Check sheet for the modelled part. Datum: model origin and axes. Units: mm. Round coordinates to 2 decimals unless told otherwise and drop trailing zeros. Loops run counter-clockwise (first coordinate to the right, second up) from the corner with the lowest first, then second, coordinate; pieces in that order, holes last. Notation, with made-up numbers: (-30, -3) - (6, -3) arc R24 ccw to (6, 10) - close; hole circle Ø5 at (65.25, 78). An arc over 180 degrees is marked (long way). Put each result on its own line as item: value. Start each with the question number.
Item 1: Draft check along Z on faces 1 (the flat face through (-71, 0, -56)), 2 (the cylindrical face through (-93.08, 1.01, -87.19)). Enter one of: pulls with the +Z half, pulls with the -Z half, needs draft (parallel to the pull), parting line crosses it, or undercut.
Item 2: Material ranges on line 1 along X through (y, z) = (1.3, -89.5); line 2 along X through (y, z) = (0.4, -105); line 3 along X through (y, z) = (1.3, -90), recorded low to high.
Item 3: Section check D-D, the plane y = 1.3. Give the number of separate pieces and of enclosed holes in the cut face, and give its area (3 significant figures).
Item 4: Section check B-B, the plane z = -90. Record the cut outline in (x, y), and give its area (3 significant figures).
Item 5: Section check A-A, the plane x = -5. Record the cut outline in (y, z), and give its area (3 significant figures).
Item 6: Section check C-C, the plane z = -105. Record the cut outline in (x, y), and give its area (3 significant figures).
Item 7: Gauge pin test, flat ends, axial feed: pin 1 Ø5.5 at (x, z) = (-135, -105) entering from +Y; pin 2 Ø4 at (x, z) = (-70, -105) entering from +Y. Record the tip position at first contact, or that the pin passes through.
from build123d import *

# Parameters (mm, degrees)
BOTTOM_PLATE_W                       = 140
BOTTOM_PLATE_H                       = 110
BOTTOM_PLATE_EXT_DEPTH               = 2
MIDDLE_ROW_R                         = 6
MIDDLE_ROW_CUT_DEPTH                 = 179.056170912
TOP_ROW_R                            = 6.1
TOP_ROW_CUT_DEPTH                    = 179.056170912
BOTTOM_ROW_R                         = 3.55
BOTTOM_ROW_R_2                       = 6
BOTTOM_ROW_CUT_DEPTH                 = 179.056170912
PLATE_SCREWS_R                       = 1.65
PLATE_SCREWS_CUT_DEPTH               = 179.056170912
PLATE_SCREW_HEAD_R                   = 2.8
PLATE_SCREW_HEAD_CUT_DEPTH           = 2
PLATE_SCREW_HEAD_CUT_DRAFT           = -45
PLATE_SCREW_HEAD_CUT_PROFILE_2_DEPTH = 2
PLATE_SCREW_HEAD_CUT_PROFILE_2_DRAFT = -45
PLATE_SCREW_HEAD_CUT_PROFILE_3_DEPTH = 2
PLATE_SCREW_HEAD_CUT_PROFILE_3_DRAFT = -45
PLATE_SCREW_HEAD_CUT_PROFILE_4_DEPTH = 2
PLATE_SCREW_HEAD_CUT_PROFILE_4_DRAFT = -45
PLATE_SCREW_HEAD_CUT_PROFILE_5_DEPTH = 2
PLATE_SCREW_HEAD_CUT_PROFILE_5_DRAFT = -45
PLATE_SCREW_HEAD_CUT_PROFILE_6_DEPTH = 2
PLATE_SCREW_HEAD_CUT_PROFILE_6_DRAFT = -45
FILLET1_R                            = 2
FILLET2_R                            = 2
FILLET3_R                            = 2
FILLET4_R                            = 2


with BuildPart() as part:
    # Bottom Plate → Bottom Plate EXT (new body)
    with BuildSketch(Plane(origin=(0, 0, 0), x_dir=(1, 0, 0), z_dir=(0, 1, 0))):
        with Locations((-70, 55)):
            Rectangle(BOTTOM_PLATE_W, BOTTOM_PLATE_H)
    extrude(amount=BOTTOM_PLATE_EXT_DEPTH)

    # Middle Row → Middle Row Cut (cut, through all)
    with BuildSketch(Plane(origin=(0, 2, 0), x_dir=(1, 0, 0), z_dir=(0, 1, 0))):
        with Locations(Location((-123, 55, 0), (0, 0, 270))):
            Circle(MIDDLE_ROW_R)
        with Locations(Location((-87.666666667, 55, 0), (0, 0, 270))):
            Circle(MIDDLE_ROW_R)
        with Locations(Location((-52.333333333, 55, 0), (0, 0, 270))):
            Circle(MIDDLE_ROW_R)
        with Locations(Location((-17, 55, 0), (0, 0, 270))):
            Circle(MIDDLE_ROW_R)
    extrude(amount=-MIDDLE_ROW_CUT_DEPTH, mode=Mode.SUBTRACT)

    # Top Row → Top Row Cut (cut, through all)
    with BuildSketch(Plane(origin=(0, 2, 0), x_dir=(1, 0, 0), z_dir=(0, 1, 0))):
        with Locations(Location((-123, 90, 0), (0, 0, 270))):
            Circle(TOP_ROW_R)
        with Locations(Location((-87.666666667, 90, 0), (0, 0, 270))):
            Circle(TOP_ROW_R)
        with Locations(Location((-52.333333333, 90, 0), (0, 0, 270))):
            Circle(TOP_ROW_R)
        with Locations(Location((-17, 90, 0), (0, 0, 270))):
            Circle(TOP_ROW_R)
    extrude(amount=-TOP_ROW_CUT_DEPTH, mode=Mode.SUBTRACT)

    # Bottom Row → Bottom Row Cut (cut, through all)
    with BuildSketch(Plane(origin=(0, 2, 0), x_dir=(1, 0, 0), z_dir=(0, 1, 0))):
        with Locations(Location((-87.666666667, 20, 0), (0, 0, 270))):
            Circle(BOTTOM_ROW_R)
        with Locations(Location((-52.333333333, 20, 0), (0, 0, 270))):
            Circle(BOTTOM_ROW_R)
        with Locations(Location((-17, 20, 0), (0, 0, 270))):
            Circle(BOTTOM_ROW_R)
        with Locations(Location((-123, 20, 0), (0, 0, 270))):
            Circle(BOTTOM_ROW_R_2)
    extrude(amount=-BOTTOM_ROW_CUT_DEPTH, mode=Mode.SUBTRACT)

    # Plate Screws → Plate Screws Cut (cut, through all)
    with BuildSketch(Plane(origin=(0, 2, 0), x_dir=(1, 0, 0), z_dir=(0, 1, 0))):
        with Locations(Location((-135, 105, 0), (0, 0, 270))):
            Circle(PLATE_SCREWS_R)
        with Locations(Location((-5, 105, 0), (0, 0, 270))):
            Circle(PLATE_SCREWS_R)
        with Locations(Location((-5, 5, 0), (0, 0, 270))):
            Circle(PLATE_SCREWS_R)
        with Locations(Location((-135, 5, 0), (0, 0, 270))):
            Circle(PLATE_SCREWS_R)
        with Locations(Location((-70, 105, 0), (0, 0, 270))):
            Circle(PLATE_SCREWS_R)
        with Locations(Location((-70, 5, 0), (0, 0, 90))):
            Circle(PLATE_SCREWS_R)
    extrude(amount=-PLATE_SCREWS_CUT_DEPTH, mode=Mode.SUBTRACT)


with BuildPart() as plate_screw_head_cut_tool:
    # Plate Screw Head → Plate Screw Head Cut (with draft: the straight prism first)
    with BuildSketch(Plane(origin=(0, 2, 0), x_dir=(1, 0, 0), z_dir=(0, 1, 0))):
        with Locations((-135, 105)):
            Circle(PLATE_SCREW_HEAD_R)
    extrude(amount=-PLATE_SCREW_HEAD_CUT_DEPTH)
    # Plate Screw Head Cut: the draft: its side faces are tilted about the plane it starts from
    plate_screw_head_cut_sides = [plate_screw_head_cut_tool.faces().sort_by_distance(p)[0] for p in [
        (-137.8, 1, -105),
    ]]
    draft(plate_screw_head_cut_sides, Plane(origin=(0, 2, 0), x_dir=(1, 0, 0), z_dir=(0, 1, 0)), PLATE_SCREW_HEAD_CUT_DRAFT)


with BuildPart() as part_1:
    add(part.part)

    # Plate Screw Head Cut: cut by plate_screw_head_cut_tool
    add(plate_screw_head_cut_tool.part, mode=Mode.SUBTRACT)


with BuildPart() as plate_screw_head_cut_profile_2_tool:
    # Plate Screw Head → Plate Screw Head Cut profile 2 (with draft: the straight prism first)
    with BuildSketch(Plane(origin=(0, 2, 0), x_dir=(1, 0, 0), z_dir=(0, 1, 0))):
        with Locations((-5, 105)):
            Circle(PLATE_SCREW_HEAD_R)
    extrude(amount=-PLATE_SCREW_HEAD_CUT_PROFILE_2_DEPTH)
    # Plate Screw Head Cut profile 2: the draft: its side faces are tilted about the plane it starts from
    plate_screw_head_cut_profile_2_sides = [plate_screw_head_cut_profile_2_tool.faces().sort_by_distance(p)[0] for p in [
        (-7.8, 1, -105),
    ]]
    draft(plate_screw_head_cut_profile_2_sides, Plane(origin=(0, 2, 0), x_dir=(1, 0, 0), z_dir=(0, 1, 0)), PLATE_SCREW_HEAD_CUT_PROFILE_2_DRAFT)


with BuildPart() as part_2:
    add(part_1.part)

    # Plate Screw Head Cut profile 2: cut by plate_screw_head_cut_profile_2_tool
    add(plate_screw_head_cut_profile_2_tool.part, mode=Mode.SUBTRACT)


with BuildPart() as plate_screw_head_cut_profile_3_tool:
    # Plate Screw Head → Plate Screw Head Cut profile 3 (with draft: the straight prism first)
    with BuildSketch(Plane(origin=(0, 2, 0), x_dir=(1, 0, 0), z_dir=(0, 1, 0))):
        with Locations((-5, 5)):
            Circle(PLATE_SCREW_HEAD_R)
    extrude(amount=-PLATE_SCREW_HEAD_CUT_PROFILE_3_DEPTH)
    # Plate Screw Head Cut profile 3: the draft: its side faces are tilted about the plane it starts from
    plate_screw_head_cut_profile_3_sides = [plate_screw_head_cut_profile_3_tool.faces().sort_by_distance(p)[0] for p in [
        (-7.8, 1, -5),
    ]]
    draft(plate_screw_head_cut_profile_3_sides, Plane(origin=(0, 2, 0), x_dir=(1, 0, 0), z_dir=(0, 1, 0)), PLATE_SCREW_HEAD_CUT_PROFILE_3_DRAFT)


with BuildPart() as part_3:
    add(part_2.part)

    # Plate Screw Head Cut profile 3: cut by plate_screw_head_cut_profile_3_tool
    add(plate_screw_head_cut_profile_3_tool.part, mode=Mode.SUBTRACT)


with BuildPart() as plate_screw_head_cut_profile_4_tool:
    # Plate Screw Head → Plate Screw Head Cut profile 4 (with draft: the straight prism first)
    with BuildSketch(Plane(origin=(0, 2, 0), x_dir=(1, 0, 0), z_dir=(0, 1, 0))):
        with Locations((-135, 5)):
            Circle(PLATE_SCREW_HEAD_R)
    extrude(amount=-PLATE_SCREW_HEAD_CUT_PROFILE_4_DEPTH)
    # Plate Screw Head Cut profile 4: the draft: its side faces are tilted about the plane it starts from
    plate_screw_head_cut_profile_4_sides = [plate_screw_head_cut_profile_4_tool.faces().sort_by_distance(p)[0] for p in [
        (-137.8, 1, -5),
    ]]
    draft(plate_screw_head_cut_profile_4_sides, Plane(origin=(0, 2, 0), x_dir=(1, 0, 0), z_dir=(0, 1, 0)), PLATE_SCREW_HEAD_CUT_PROFILE_4_DRAFT)


with BuildPart() as part_4:
    add(part_3.part)

    # Plate Screw Head Cut profile 4: cut by plate_screw_head_cut_profile_4_tool
    add(plate_screw_head_cut_profile_4_tool.part, mode=Mode.SUBTRACT)


with BuildPart() as plate_screw_head_cut_profile_5_tool:
    # Plate Screw Head → Plate Screw Head Cut profile 5 (with draft: the straight prism first)
    with BuildSketch(Plane(origin=(0, 2, 0), x_dir=(1, 0, 0), z_dir=(0, 1, 0))):
        with Locations((-70, 105)):
            Circle(PLATE_SCREW_HEAD_R)
    extrude(amount=-PLATE_SCREW_HEAD_CUT_PROFILE_5_DEPTH)
    # Plate Screw Head Cut profile 5: the draft: its side faces are tilted about the plane it starts from
    plate_screw_head_cut_profile_5_sides = [plate_screw_head_cut_profile_5_tool.faces().sort_by_distance(p)[0] for p in [
        (-72.8, 1, -105),
    ]]
    draft(plate_screw_head_cut_profile_5_sides, Plane(origin=(0, 2, 0), x_dir=(1, 0, 0), z_dir=(0, 1, 0)), PLATE_SCREW_HEAD_CUT_PROFILE_5_DRAFT)


with BuildPart() as part_5:
    add(part_4.part)

    # Plate Screw Head Cut profile 5: cut by plate_screw_head_cut_profile_5_tool
    add(plate_screw_head_cut_profile_5_tool.part, mode=Mode.SUBTRACT)


with BuildPart() as plate_screw_head_cut_profile_6_tool:
    # Plate Screw Head → Plate Screw Head Cut profile 6 (with draft: the straight prism first)
    with BuildSketch(Plane(origin=(0, 2, 0), x_dir=(1, 0, 0), z_dir=(0, 1, 0))):
        with Locations((-70, 5)):
            Circle(PLATE_SCREW_HEAD_R)
    extrude(amount=-PLATE_SCREW_HEAD_CUT_PROFILE_6_DEPTH)
    # Plate Screw Head Cut profile 6: the draft: its side faces are tilted about the plane it starts from
    plate_screw_head_cut_profile_6_sides = [plate_screw_head_cut_profile_6_tool.faces().sort_by_distance(p)[0] for p in [
        (-72.8, 1, -5),
    ]]
    draft(plate_screw_head_cut_profile_6_sides, Plane(origin=(0, 2, 0), x_dir=(1, 0, 0), z_dir=(0, 1, 0)), PLATE_SCREW_HEAD_CUT_PROFILE_6_DRAFT)


with BuildPart() as part_6:
    add(part_5.part)

    # Plate Screw Head Cut profile 6: cut by plate_screw_head_cut_profile_6_tool
    add(plate_screw_head_cut_profile_6_tool.part, mode=Mode.SUBTRACT)

    # Fillet1
    fillet1_edges = [part_6.edges().sort_by_distance(p)[0] for p in [
        (-140, 1, -110),
    ]]
    fillet(fillet1_edges, radius=FILLET1_R)

    # Fillet2
    fillet2_edges = [part_6.edges().sort_by_distance(p)[0] for p in [
        (0, 1, -110),
    ]]
    fillet(fillet2_edges, radius=FILLET2_R)

    # Fillet3
    fillet3_edges = [part_6.edges().sort_by_distance(p)[0] for p in [
        (0, 1, 0),
    ]]
    fillet(fillet3_edges, radius=FILLET3_R)

    # Fillet4
    fillet4_edges = [part_6.edges().sort_by_distance(p)[0] for p in [
        (-140, 1, 0),
    ]]
    fillet(fillet4_edges, radius=FILLET4_R)


solid = part_6.part
Check result:
1. face 1: needs draft
1. face 2: undercut
2. line 1: -140 to -129.08, -116.92 to -93.75, -81.59 to -58.41, -46.25 to -23.08, -10.92 to 0
2. line 2: -140 to -136.65, -133.35 to -71.65, -68.35 to -6.65, -3.35 to 0
2. line 3: -140 to -129.1, -116.9 to -93.77, -81.57 to -58.43, -46.23 to -23.1, -10.9 to 0
3. separate pieces: 1
3. enclosed holes: 18
3. area: 14,200 mm²
4. outline: (-140, 0) - (-129.1, 0) - (-129.1, 2) - (-140, 2) - close; (-116.9, 0) - (-93.77, 0) - (-93.77, 2) - (-116.9, 2) - close; (-81.57, 0) - (-58.43, 0) - (-58.43, 2) - (-81.57, 2) - close; (-46.23, 0) - (-23.1, 0) - (-23.1, 2) - (-46.23, 2) - close; (-10.9, 0) - (0, 0) - (0, 2) - (-10.9, 2) - close
4. area: 182 mm²
5. outline: (0, -110) - (2, -110) - (2, -107.8) - (0.85, -106.65) - (0, -106.65) - close; (0, -103.35) - (0.85, -103.35) - (2, -102.2) - (2, -7.8) - (0.85, -6.65) - (0, -6.65) - close; (0, -3.35) - (0.85, -3.35) - (2, -2.2) - (2, 0) - (0, 0) - close
5. area: 204 mm²
6. outline: (-140, 0) - (-136.65, 0) - (-136.65, 0.85) - (-137.8, 2) - (-140, 2) - close; (-133.35, 0) - (-71.65, 0) - (-71.65, 0.85) - (-72.8, 2) - (-132.2, 2) - (-133.35, 0.85) - close; (-68.35, 0) - (-6.65, 0) - (-6.65, 0.85) - (-7.8, 2) - (-67.2, 2) - (-68.35, 0.85) - close; (-3.35, 0) - (0, 0) - (0, 2) - (-2.2, 2) - (-3.35, 0.85) - close
6. area: 256 mm²
7. pin 1: y = 1.95
7. pin 2: y = 1.2
